Here's how the part is built. I have some questions about the finished solid (model axes, mm). Give positions to 0.01 mm unless a question says otherwise; leave off trailing zeros. Write each loop counter-clockwise with the first axis right and the second up, starting at its lowest first coordinate (ties: lowest second). Pieces come first, ordered by that corner, then holes. Notation, with made-up numbers: (22.5, 54.25) -> (64.5, 54.25) arc R17 cw to (64.5, 84.25) -> close; hole circle Ø10 at (86.25, 56). An arc over 180 degrees is marked (long way). Use one line per item in the form item = value.
Autodesk Inventor part; units mm, degrees
ref_plane "YZ Plane" through (0, 0, 0) normal (1, 0, 0) x (0, 1, 0)
ref_plane "XZ Plane" through (0, 0, 0) normal (0, 1, 0) x (-1, 0, 0)
ref_plane "XY Plane" through (0, 0, 0) normal (0, 0, 1) x (1, 0, 0)
sketch "Szkic1" plane through (0, 0, 0) normal (0, 0, 1) x (1, 0, 0)
  circle A0 centre (0, 0) radius 43.5 construction
  line L0 (0, 43.5) -> (2.5, 43.5) construction
  line L1 (2.5, 43.5) -> (2.5, 75.9975) construction
  line L2 (2.5, 75.9975) -> (0, 75.9975) construction
  line L3 (0, 75.9975) -> (0, 43.5) construction
  line L4 (0, -43.5) -> (2.5, -43.5) construction
  line L5 (2.5, -43.5) -> (2.5, -75.9975) construction
  line L6 (2.5, -75.9975) -> (0, -75.9975) construction
  line L7 (43.5, 0) -> (75.9975, 0) construction
  line L8 (75.9975, 0) -> (75.9975, 2.5) construction
  line L9 (75.9975, 2.5) -> (43.5, 2.5) construction
  line L10 (43.5, 2.5) -> (43.5, 0) construction
  line L11 (43.5, 0) -> (75.9975, 0) construction
  line L12 (75.9975, 0) -> (75.9975, -2.5) construction
  line L13 (75.9975, -2.5) -> (43.5, -2.5) construction
  line L14 (43.5, -2.5) -> (43.5, 0) construction
  line L15 (0, 43.5) -> (-2.5, 43.5) construction
  line L16 (-2.5, 43.5) -> (-2.5, 75.9975) construction
  line L17 (-2.5, 75.9975) -> (0, 75.9975) construction
  line L18 (0, 75.9975) -> (0, 43.5) construction
  line L19 (0, -43.5) -> (-5, -43.5) construction
  line L20 (-5, -43.5) -> (-5, -75.9975) construction
  line L21 (-5, -75.9975) -> (-2.5, -75.9975) construction
  line L22 (-43.5, 0) -> (-75.9975, 0) construction
  line L23 (-75.9975, 0) -> (-75.9975, -2.5) construction
  line L24 (-75.9975, -2.5) -> (-43.5, -2.5) construction
  line L25 (-43.5, -2.5) -> (-43.5, 0) construction
  line L26 (-43.5, 0) -> (-75.9975, 0) construction
  line L27 (-75.9975, 0) -> (-75.9975, 2.5) construction
  line L28 (-75.9975, 2.5) -> (-43.5, 2.5) construction
  line L29 (-43.5, 2.5) -> (-43.5, 0) construction
  arc A1 (2.5, -43.4281) -> (43.4281, -2.5) centre (0, 0) ccw
  arc A2 (43.4281, 2.5) -> (2.5, 43.4281) centre (0, 0) ccw
  arc A3 (-43.4281, -2.5) -> (-5, -43.2117) centre (0, 0) ccw
  arc A4 (-2.5, 43.4281) -> (-43.4281, 2.5) centre (0, 0) ccw
  line L30 (-2.5, 43.4281) -> (-2.5, 75.9975)
  line L31 (-2.5, 75.9975) -> (2.5, 75.9975)
  line L32 (2.5, 75.9975) -> (2.5, 43.4281)
  line L33 (43.4281, 2.5) -> (75.9975, 2.5)
  line L34 (75.9975, 2.5) -> (75.9975, -2.5)
  line L35 (75.9975, -2.5) -> (43.4281, -2.5)
  line L36 (2.5, -43.4281) -> (2.5, -75.9975)
  line L37 (2.5, -75.9975) -> (-5, -75.9975)
  line L38 (-5, -75.9975) -> (-5, -43.2117)
  line L39 (-43.4281, -2.5) -> (-75.9975, -2.5)
  line L40 (-75.9975, -2.5) -> (-75.9975, 2.5)
  line L41 (-75.9975, 2.5) -> (-43.4281, 2.5)
  dimension "d0" = 87
  dimension "d1" = 2.5
  dimension "d3" = 2.5
  dimension "d6" = 2.5
  dimension "d7" = 2.5
  dimension "d8" = 2.5
  dimension "d9" = 2.5
  dimension "d11" = 2.5
  dimension "d12" = 2.5
  dimension "d15" = 75.9975
  dimension "d16" = 75.9975
  dimension "d17" = 75.9975
  dimension "d19" = 75.9975
extrude "Wyciągnięcie proste1" add sketch "Szkic1" along normal blind 6
equation "\"d1\" = d11"
equation "\"d3\" = d11"
equation "\"d6\" = d11"
equation "\"d7\" = d11"
equation "\"d8\" = d11"
equation "\"d9\" = d11"
equation "\"d12\" = d11"
properties part number "Zamek_II_klucz"
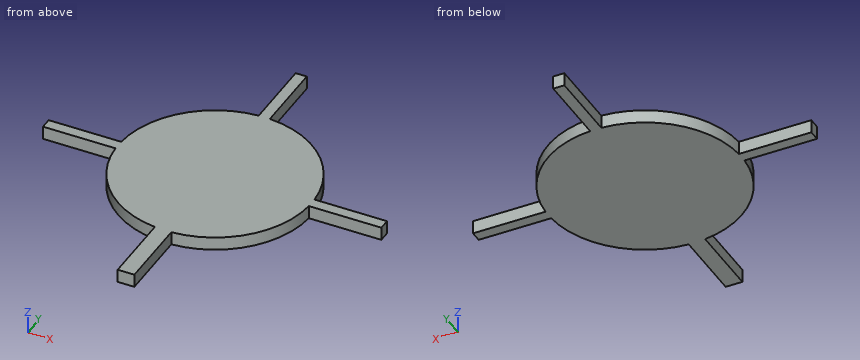
Q1. I want a section at A-A, the plane z = 0.95. Write out the boundary of the cut face in (x, y).
Result set:
outline = (-76, -2.5) -> (-43.43, -2.5) arc R43.5 ccw to (-5, -43.21) -> (-5, -76) -> (2.5, -76) -> (2.5, -43.43) arc R43.5 ccw to (43.43, -2.5) -> (76, -2.5) -> (76, 2.5) -> (43.43, 2.5) arc R43.5 ccw to (2.5, 43.43) -> (2.5, 76) -> (-2.5, 76) -> (-2.5, 43.43) arc R43.5 ccw to (-43.43, 2.5) -> (-76, 2.5) -> close
Q2. If I drill on line 1 along X through (y, z) = (62.5, 0.8); line 2 along X through (y, z) = (3, 4.25), over which ranges is the centre line in solid material (lowest first)? Write a range as from..to.
Result set:
line_1 = -2.5..2.5
line_2 = -43.4..43.4
Q3. I want a section at B-B, the plane y = 50. Write out the boundary of the cut face in (x, z).
Result set:
outline = (-2.5, 0) -> (2.5, 0) -> (2.5, 6) -> (-2.5, 6) -> close
Q4. Will these pins go through, and if not, where does the flat tip stop? pin 1 Ø2 at (x, z) = (19.5, 4.5) entering from +Y; pin 2 Ø1.8 at (x, z) = (-66.5, 4.5) entering from +Y; pin 3 Ø1 at (y, z) = (-37.5, 5) entering from -X; pin 4 Ø12 at (x, y) = (27.5, -26.5) entering from -Z.
Result set:
pin_1 = 39.37
pin_2 = 2.5
pin_3 = -22.87
pin_4 = 0
